from build123d import *

# Parameters (mm, degrees)
F0_R     = 3
F1_DEPTH = 10
F1_TAPER = -20
F2_R     = 2
F3_R     = 2
F4_DEPTH = 3


with BuildPart() as f1:
    # F0 (on Top) → F1 (new body)
    with BuildSketch(Plane.XY):
        Circle(F0_R)
    extrude(amount=F1_DEPTH, taper=F1_TAPER)

    # F2
    f2_edges = [f1.edges().sort_by_distance(p)[0] for p in [
        (-6.639702, 0, 10),
    ]]
    fillet(f2_edges, radius=F2_R)

    # F3 (on face) → F4 (join)
    with BuildSketch(Plane(origin=(0, 0, 0), x_dir=(1, 0, 0), z_dir=(0, 0, -1))):
        Circle(F3_R)
    extrude(amount=F4_DEPTH)


solid = f1.part
Can you work these out from the model? Positions are in its coordinate system, mm. A direction names the side the tool comes from. Coordinates: 2 decimals unless noted, no trailing zeros. Loops run counter-clockwise (first coordinate to the right, second up) from the corner with the lowest first, then second, coordinate; pieces in that order, holes last. Notation, with made-up numbers: (58.25, 30.25) - (95.25, 30.25) arc R24 cw to (95.25, 55.25) - close; hole circle Ø8 at (70, -18). An arc over 180 degrees is marked (long way). Put each result on its own line as item: value. Start each with the question number.
Item 1: Suppose I cut it at A-A (x = 0). Please give me the cut outline in (y, z).
Item 2: If I drill on line 1 along Z through (x, y) = (-1.5, -2); line 2 along X through (y, z) = (1, 6.5); line 3 along Y through (x, z) = (5.25, 7.5), over which ranges is the centre line in solid material (lowest first)?
Item 3: Suppose I cut it at C-C (z = 6). Please give me the cut outline in (x, y).
Item 4: Which directions (+Z, -Z, +X, -X, +Y, -Y) give clear straight access to the entire face, cutting with the end or side of a thin tool? Please do faces 1 (the face through (0, 2, -1)), 2 (the face through (0, 0, 10)).
Item 5: For pin 1 (2 mm diameter, centred on y = -4, z = -1, fed in from +X); pin 2 (1.5 mm diameter, centred on y = -3, z = 7, fed in from +X); pin 3 (3 mm diameter, centred on x = 1, y = -4, fed in from -Z); pin 4 (5 mm diameter, centred on y = 1, z = 1, fed in from -X), each with a flat end and sliding along its axis, tell me the tip position at first contact or that it passes through.
Item 6: Suppose I cut it at B-B (z = -0.75). Please give me the cut outline in (x, y).
Here are the results:
1. outline: (-5.66, 7.32) - (-3, 0) - (-2, 0) - (-2, -3) - (2, -3) - (2, 0) - (3, 0) - (5.66, 7.32) arc R2 ccw to (3.78, 10) - (-3.78, 10) arc R2 ccw to start
2. line 1: 0 to 10
2. line 2: -5.27 to 5.27
2. line 3: -2.27 to 2.27
3. outline: circle Ø10.37 at (0, 0)
4. face 1: -Z
4. face 2: +Z, +X, -X, +Y, -Y
5. pin 1: through
5. pin 2: x = 5.18
5. pin 3: z = 0
5. pin 4: x = -4.23
6. outline: circle Ø4 at (0, 0)
